```python
from build123d import *

# Parameters (mm, degrees)
SKETCH1_W                       = 2
SKETCH1_H                       = 2
BOSS_EXTRUDE1_DEPTH             = 20
BOSS_EXTRUDE2_REACH             = 22.05
SKETCH2_R                       = 1.5
BOSS_EXTRUDE2_DIRECTION_2_REACH = 22.05
CUT_EXTRUDE1_DEPTH              = 21.081085628
CUT_EXTRUDE1_DEPTH_BACK         = 21.081085628
SKETCH3_R                       = 0.75
SKETCH4_W                       = 8
SKETCH4_H                       = 30
BOSS_EXTRUDE4_DEPTH             = 2.81
CUT_EXTRUDE3_DEPTH              = 41.78622439
LPATTERN1_COUNT                 = 14
LPATTERN1_PITCH                 = 2
LPATTERN1_COL_COUNT             = 2
LPATTERN1_COL_PITCH             = 2
FILLET2_R                       = 0.5


with BuildPart() as part:
    # Sketch1 → Boss-Extrude1 (new body)
    with BuildSketch(Plane.XY):
        Rectangle(SKETCH1_W, SKETCH1_H)
    extrude(amount=BOSS_EXTRUDE1_DEPTH)

    # Boss-Extrude2: up to this face of the body (flat: up to its plane)
    boss_extrude2_end = Plane(part.part.faces().sort_by_distance((1, 0, 10))[0])
    # Sketch2 → Boss-Extrude2 (add, up to the picked face)
    with BuildSketch(Plane(origin=(0, 0, 0), x_dir=(0, 0, -1), z_dir=(1, 0, 0)), mode=Mode.PRIVATE) as boss_extrude2_sk1:
        Circle(SKETCH2_R)
    boss_extrude2_tool1 = split(extrude(boss_extrude2_sk1.sketch, amount=BOSS_EXTRUDE2_REACH, mode=Mode.PRIVATE), bisect_by=boss_extrude2_end, keep=Keep.BOTH, mode=Mode.PRIVATE)
    add(boss_extrude2_tool1.solids().sort_by(Axis((0, 0, 0), (1, 0, 0)))[0])

    # Boss-Extrude2 direction 2: up to this face of the body (flat: up to its plane)
    boss_extrude2_direction_2_end = Plane(part.part.faces().sort_by_distance((-1, 0, 10))[0])
    # Sketch2 → Boss-Extrude2 direction 2 (add, up to the picked face)
    with BuildSketch(Plane(origin=(0, 0, 0), x_dir=(0, 0, -1), z_dir=(1, 0, 0)), mode=Mode.PRIVATE) as boss_extrude2_direction_2_sk1:
        Circle(SKETCH2_R)
    boss_extrude2_direction_2_tool1 = split(extrude(boss_extrude2_direction_2_sk1.sketch, amount=-BOSS_EXTRUDE2_DIRECTION_2_REACH, mode=Mode.PRIVATE), bisect_by=boss_extrude2_direction_2_end, keep=Keep.BOTH, mode=Mode.PRIVATE)
    add(boss_extrude2_direction_2_tool1.solids().sort_by(Axis((0, 0, 0), (-1, 0, 0)))[0])

    # Sketch3 → Cut-Extrude1 (cut, two sides: drawn at the far end of the back side and taken through both)
    with BuildSketch(Plane(origin=(0, 0, 0), x_dir=(0, 0, -1), z_dir=(1, 0, 0)).offset(-CUT_EXTRUDE1_DEPTH_BACK)):
        Circle(SKETCH3_R)
    extrude(amount=CUT_EXTRUDE1_DEPTH + CUT_EXTRUDE1_DEPTH_BACK, mode=Mode.SUBTRACT)

    # Sketch4 → Boss-Extrude4 (add)
    with BuildSketch(Plane(origin=(0, 1, 0), x_dir=(1, 0, 0), z_dir=(0, 1, 0))):
        with Locations((-3, -25)):
            Rectangle(SKETCH4_W, SKETCH4_H)
    extrude(amount=BOSS_EXTRUDE4_DEPTH)

    # Sketch9 → Cut-Extrude3 (cut, symmetric)
    with BuildSketch(Plane(origin=(0, 0, 0), x_dir=(0, 0, -1), z_dir=(1, 0, 0))):
        with BuildLine():
            ThreePointArc((-38.315329673, 4.397253742), (-37.483653354, 3.101788083), (-37.158231048, 1.597122972))
            ThreePointArc((-37.158231048, 1.597122972), (-36.989658323, 1.6), (-36.821085598, 1.597122972))
            ThreePointArc((-36.821085598, 1.597122972), (-36.495663293, 3.101788083), (-35.663986973, 4.397253742))
            ThreePointArc((-35.663986973, 4.397253742), (-36.989658323, 4.51), (-38.315329673, 4.397253742))
        make_face()
    cut_extrude3 = extrude(amount=CUT_EXTRUDE3_DEPTH, both=True, mode=Mode.SUBTRACT)

    # LPattern1: Cut-Extrude3 ×14
    with Locations(*[(0, 0, -i * LPATTERN1_PITCH) for i in range(1, LPATTERN1_COUNT)]):
        add(cut_extrude3, mode=Mode.SUBTRACT)

    # LPattern1 col: Cut-Extrude3 ×2
    with Locations(*[(0, 0, i * LPATTERN1_COL_PITCH) for i in range(1, LPATTERN1_COL_COUNT)]):
        add(cut_extrude3, mode=Mode.SUBTRACT)

    # Fillet2
    fillet2_edges = [part.edges().sort_by_distance(p)[0] for p in [
        (-1, -1, 10.559016994),
        (1, -1, 10.559016994),
        (1, 1, 5.559016994),
        (-1, 1, 5.559016994),
        (0, -1, 20),
        (0, 1, 20),
    ]]
    fillet(fillet2_edges, radius=FILLET2_R)


solid = part.part
```
Geometry check sheet. Reference: the model listing, model coordinates, mm. A direction names the side the tool comes from. Coordinates: 2 decimals unless noted, no trailing zeros. Order: outer loops, then holes, each group sorted by start corner. A loop starts at its lowest first (then second) coordinate and runs counter-clockwise, first axis right, second up. Notation, with made-up numbers: (20.25, 39.5) - (48.25, 39.5) arc R25 ccw to (48.25, 66.5) - close; hole circle Ø4 at (-30.5, 11). An arc over 180 degrees is marked (long way). Answer in a Markdown table with one row per item. Add a question column.
1. Draft check along Z on faces 1 (the face through (0, 1, 5)), 2 (the face through (-3, 1, 25)), 3 (the face through (0, 0, 20)). Enter one of: +Z half, -Z half, draft (parallel to the pull), parting line (faces both ways), or undercut.
2. Access from +Z, -Z, +X, -X, +Y, -Y to the whole of each face (thin tool, end or side, straight path). Record for faces 4 (the face through (0, -1, 10)), 5 (the face through (-2.944, 2.767, 11.361)), 6 (the face through (1, 2, 20)).
3. Section check A-A (z = 0). Enter the section's corners in (x, y), plus the area to 3 significant figures.
4. Section check B-B (y = 0). Enter the section's corners in (x, z), plus the area to 3 significant figures.
5. Gauge pin test, flat ends, axial feed: pin 1 Ø4 at (x, z) = (0, 32) entering from -Y; pin 2 Ø1.5 at (y, z) = (0.5, 7.5) entering from -X; pin 3 Ø0.8 at (x, z) = (0, 14.5) entering from -Y. Record the tip position at first contact, or that the pin passes through.
6. Section check D-D (y = 3.15). Give the number of separate pieces and of enclosed holes in the cut face, plus the area to 3 significant figures.
7. Section check C-C (z = 17.5). Enter the section's corners in (x, y), plus the area to 3 significant figures.
8. Material ranges on L1, parallel to Z at x = 0.5, y = 0; L2, parallel to Y at x = -0.35, z = 0; L3, parallel to Y at x = -3, z = 15, recorded low to high. Write a range as [from, to].
Data:
| question | item | result |
|---|---|---|
| 1 | face 1 | undercut |
| 1 | face 2 | draft |
| 1 | face 3 | +Z half |
| 2 | face 4 | +Z, +X, -X, -Y |
| 2 | face 5 | +X, -X, +Y |
| 2 | face 6 | +Z, -Z, +X, +Y, -Y |
| 3 | outline | (-1, -1.5) - (1, -1.5) - (1, -0.75) - (-1, -0.75) - close; (-1, 0.75) - (1, 0.75) - (1, 1.5) - (-1, 1.5) - close |
| 3 | area | 3.00 mm² |
| 4 | outline | (-1, -1.5) - (1, -1.5) - (1, -0.75) - (-1, -0.75) - close; (-1, 0.75) - (1, 0.75) - (1, 20) - (-1, 20) - close |
| 4 | area | 40.0 mm² |
| 5 | pin 1 | stops at y = 1 |
| 5 | pin 2 | stops at x = -1 |
| 5 | pin 3 | stops at y = -1 |
| 6 | separate pieces | 16 |
| 6 | enclosed holes | 0 |
| 6 | area | 117 mm² |
| 7 | outline | (-7, 1) - (-1, 1) - (-1, -0.5) arc R0.5 ccw to (-0.5, -1) - (0.5, -1) arc R0.5 ccw to (1, -0.5) - (1, 3.14) - (-7, 3.14) - close |
| 7 | area | 21.0 mm² |
| 8 | L1 | z = [-1.5, -0.75], [0.75, 20] |
| 8 | L2 | y = [-1.5, -0.75], [0.75, 1.5] |
| 8 | L3 | y = [1, 1.6] |
